For this review, take the finished solid that the model builds, in its own axes (mm). A direction names the side the tool comes from. Give positions to 0.01 mm unless a question says otherwise; leave off trailing zeros. Order: outer loops, then holes, each group sorted by start corner. A loop starts at its lowest first (then second) coordinate and runs counter-clockwise, first axis right, second up. Notation, with made-up numbers: (9, -8) -> (19, -8) arc R22 cw to (19, 31) -> close; hole circle Ø9 at (20, -1.75). An arc over 180 degrees is marked (long way). Return JSON: item names as keys, results as strings. Group by question number.
1) The part is to be moulded in two halves that separate along X. For faces 1 (the face through (70, 7.3, -7.3)), 2 (the face through (-10, 1, 70)), 3 (the face through (-40, 0, 0)), say which applies: released by +X, released by -X, zero draft, split by the parting line, or undercut.
2) Add section C-C (x = 86.5). Give the boundary of the cut face in (y, z).
3) To check wall thickness, follow line 1 along X through (y, z) = (34.5, 20.5); line 2 along X through (y, z) = (7, -18.5); line 3 along Z through (x, y) = (69, 6). State the ranges of each line that lie inside material, in increasing order.
4) Add section D-D (y = 16). Give the boundary of the cut face in (x, z), then the cut area to 3 significant figures.
5) Add section B-B (z = 0). Give the boundary of the cut face in (x, y), then the cut area to 3 significant figures.
6) Insertion check: P1, Ø6, axis at y = -12.5, z = 43.5, coming from the +X side; P2, Ø3, axis at y = 29.5, z = -27, coming from the -X side; P3, Ø8, axis at x = 8, z = -28, coming from the +Y side. Each pin has a flat end and moves straight along its axis. Give the tip position at first contact, or say it passes through.
7) For faces 4 (the face through (-20, 34, 17)), 5 (the face through (89.72, -2.17, -9.76)), 6 (the face through (-10, 50, -1)), list the 3-axis set-ups (+Z, -Z, +X, -X, +Y, -Y) from which the entire face can be reached by the end or side of a thin tool; tool diameter is ignored.
8) Add section A-A (y = 0). Give the boundary of the cut face in (x, z), then the cut area to 3 significant figures.
from build123d import *

# Parameters (mm, degrees)
F0_R     = 35
F1_DEPTH = 70
F2_R     = 10
F3_DEPTH = 40
F4_W     = 100
F4_H     = 140
F4_R     = 35
F5_DEPTH = 20
F6_R     = 35
F7_DEPTH = 20


with BuildPart() as f1:
    # F0 (on Right) → F1 (new body)
    with BuildSketch(Plane.YZ):
        Circle(F0_R)
    extrude(amount=F1_DEPTH)

    # F2 (on face) → F3 (join)
    with BuildSketch(Plane.YZ.offset(70)):
        Circle(F2_R)
    extrude(amount=F3_DEPTH)

    # F4 (on face) → F5 (join)
    with BuildSketch(Plane(origin=(0, 0, 0), x_dir=(0, -1, 0), z_dir=(-1, 0, 0))):
        Rectangle(F4_W, F4_H)
        Circle(F4_R, mode=Mode.SUBTRACT)
        Circle(F4_R)
    extrude(amount=F5_DEPTH)

    # F6 (on face) → F7 (join)
    with BuildSketch(Plane(origin=(-20, 0, 0), x_dir=(0, -1, 0), z_dir=(-1, 0, 0))):
        Circle(F6_R)
    extrude(amount=F7_DEPTH)


solid = f1.part
Evaluation:
{
 "1": {"face 1": "released by +X", "face 2": "zero draft", "face 3": "released by -X"},
 "2": {"outline": "circle Ø20 at (0, 0)"},
 "3": {"line 1": "-20 to 0", "line 2": "-40 to 70", "line 3": "-34.48 to 34.48"},
 "4": {"outline": "(-40, -31.13) -> (-20, -31.13) -> (-20, -70) -> (0, -70) -> (0, -31.13) -> (70, -31.13) -> (70, 31.13) -> (0, 31.13) -> (0, 70) -> (-20, 70) -> (-20, 31.13) -> (-40, 31.13) -> close", "area": "8,400 mm^2"},
 "5": {"outline": "(-40, -35) -> (-20, -35) -> (-20, -50) -> (0, -50) -> (0, -35) -> (70, -35) -> (70, -10) -> (110, -10) -> (110, 10) -> (70, 10) -> (70, 35) -> (0, 35) -> (0, 50) -> (-20, 50) -> (-20, 35) -> (-40, 35) -> close", "area": "9,100 mm^2"},
 "6": {"P1": "x = 0", "P2": "x = -20", "P3": "y = 25.48"},
 "7": {"face 4": "-X", "face 5": "+X", "face 6": "+Z, -Z, +X, -X, +Y"},
 "8": {"outline": "(-40, -35) -> (-20, -35) -> (-20, -70) -> (0, -70) -> (0, -35) -> (70, -35) -> (70, -10) -> (110, -10) -> (110, 10) -> (70, 10) -> (70, 35) -> (0, 35) -> (0, 70) -> (-20, 70) -> (-20, 35) -> (-40, 35) -> close", "area": "9,900 mm^2"}
}
